Model file for the job. Use its own axes, mm. Round coordinates to 2 decimals unless told otherwise and drop trailing zeros. Order: outer loops, then holes, each group sorted by start corner. A loop starts at its lowest first (then second) coordinate and runs counter-clockwise, first axis right, second up. Notation, with made-up numbers: (28.25, 69.5) - (40.25, 69.5) arc R8 cw to (40.25, 82.5) - close; hole circle Ø10 at (5, 54). An arc over 180 degrees is marked (long way). Write item = value, one per line.
```python
from build123d import *

# Parameters (mm, degrees)
SKETCH1_R           = 4.3
BOSS_EXTRUDE1_DEPTH = 3


with BuildPart() as part:
    # Sketch1 → Boss-Extrude1 (new body)
    with BuildSketch(Plane.XY):
        with BuildLine():
            Line((-35.59279418, 39.784944199), (-35.59279418, -39.784944199))
            Line((-35.59279418, -39.784944199), (35.59279418, -39.784944199))
            Line((35.59279418, -39.784944199), (35.59279418, 39.784944199))
            Line((35.59279418, 39.784944199), (5, 39.784944199))
            Line((5, 39.784944199), (5, 34.7))
            ThreePointArc((5, 34.7), (0, 29.7), (-5, 34.7))
            Line((-5, 34.7), (-5, 39.784944199))
            Line((-5, 39.784944199), (-35.59279418, 39.784944199))
        make_face()
        with Locations((-26.65, -29.8)):
            Circle(SKETCH1_R, mode=Mode.SUBTRACT)
        with Locations((26.65, -29.8)):
            Circle(SKETCH1_R, mode=Mode.SUBTRACT)
        with Locations((-26.65, 29.8)):
            Circle(SKETCH1_R, mode=Mode.SUBTRACT)
        with Locations((26.65, 29.8)):
            Circle(SKETCH1_R, mode=Mode.SUBTRACT)
    extrude(amount=BOSS_EXTRUDE1_DEPTH)


solid = part.part
```
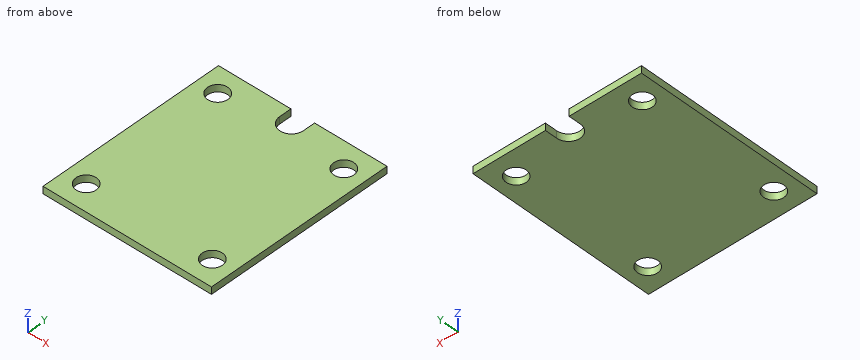
1) Wall check: line 1 along Y through (x, z) = (-26.65, 2.1); line 2 along Y through (x, z) = (28, 2.05); line 3 along Y through (x, z) = (-0.5, 2.2). Give the ranges that are in metal, low to high.
Conclusion:
line_1 = -39.78 to -34.1, -25.5 to 25.5, 34.1 to 39.78
line_2 = -39.78 to -33.88, -25.72 to 25.72, 33.88 to 39.78
line_3 = -39.78 to 29.73
2) Cut at B-B (z = 2.5). Write the cut outline in (x, y).
Conclusion:
outline = (-35.59, -39.78) - (35.59, -39.78) - (35.59, 39.78) - (5, 39.78) - (5, 34.7) arc R5 cw to (-5, 34.7) - (-5, 39.78) - (-35.59, 39.78) - close; hole circle Ø8.6 at (-26.65, -29.8); hole circle Ø8.6 at (-26.65, 29.8); hole circle Ø8.6 at (26.65, -29.8); hole circle Ø8.6 at (26.65, 29.8)
3) Cut at C-C (y = -29.8). Write the cut outline in (x, z).
Conclusion:
outline = (-35.59, 0) - (-30.95, 0) - (-30.95, 3) - (-35.59, 3) - close; (-22.35, 0) - (22.35, 0) - (22.35, 3) - (-22.35, 3) - close; (30.95, 0) - (35.59, 0) - (35.59, 3) - (30.95, 3) - close
4) Cut at D-D (x = 0). Write the cut outline in (y, z), and give its area (3 significant figures).
Conclusion:
outline = (-39.78, 0) - (29.7, 0) - (29.7, 3) - (-39.78, 3) - close
area = 208 mm^2
5) Cut at A-A (x = -26.65). Write the cut outline in (y, z).
Conclusion:
outline = (-39.78, 0) - (-34.1, 0) - (-34.1, 3) - (-39.78, 3) - close; (-25.5, 0) - (25.5, 0) - (25.5, 3) - (-25.5, 3) - close; (34.1, 0) - (39.78, 0) - (39.78, 3) - (34.1, 3) - close
